Geometry check sheet. Reference: the model listing, model coordinates, mm. A direction names the side the tool comes from. Give positions to 0.01 mm unless a question says otherwise; leave off trailing zeros. Loops run counter-clockwise (first coordinate to the right, second up) from the corner with the lowest first, then second, coordinate; pieces in that order, holes last. Notation, with made-up numbers: (49, 36) -> (92, 36) arc R22 cw to (92, 72) -> close; hole circle Ø1 at (-6.5, 81). An arc over 180 degrees is marked (long way). One line per question, with ' | ' between items.
Autodesk Inventor part; units mm, degrees
ref_plane "YZ Plane" through (0, 0, 0) normal (1, 0, 0) x (0, 1, 0)
ref_plane "XZ Plane" through (0, 0, 0) normal (0, 1, 0) x (-1, 0, 0)
ref_plane "XY Plane" through (0, 0, 0) normal (0, 0, 1) x (1, 0, 0)
sketch "スケッチ1" plane through (0, 0, 0) normal (0, 0, 1) x (1, 0, 0)
  line L0 (-5, 5) -> (5, 5)
  line L1 (5, 5) -> (5, -5)
  line L2 (5, -5) -> (-5, -5)
  line L3 (-5, -5) -> (-5, 5)
  line L4 (-5, 5) -> (5, -5) construction
  line L5 (5, 5) -> (-5, -5) construction
  point P0 (0, 0)
  dimension "d0" = 10
  dimension "d1" = 10
extrude "押し出し1" add sketch "スケッチ1" along normal blind 1
sketch "スケッチ4" plane through (0, 0, 1) normal (0, 0, 1) x (1, 0, 0)
  line L0 (-5, 5) -> (5, 5)
  line L1 (5, 5) -> (5, 6)
  line L2 (5, 6) -> (-5, 6)
  line L3 (-5, 6) -> (-5, 5)
  point P0 (0, 0)
  dimension "d11" = 1
extrude "押し出し2" add sketch "スケッチ4" against normal blind 30
sketch "スケッチ9" plane through (0, 0, 0) normal (0, 0, -1) x (-1, 0, 0)
  line L0 (-5, -5) -> (5, -5)
  line L1 (5, -5) -> (5, 5)
  line L2 (5, 5) -> (-5, 5)
  line L3 (-5, 5) -> (-5, -5)
  point P0 (0, 0)
extrude "押し出し6" add sketch "スケッチ9" along normal blind 0.5
sketch "スケッチ10" plane through (0, 0, 1) normal (0, 0, 1) x (1, 0, 0)
  circle A0 centre (0, 0) radius 1.55
  dimension "d37" = 3.1
extrude "押し出し7" cut sketch "スケッチ10" against normal blind 3
sketch "スケッチ11" plane through (-5, 5, -29) normal (0, -1, 0) x (1, 0, 0)
  line L0 (0, 0) -> (10, 0)
  line L1 (10, 0) -> (10, 28.5)
  line L2 (10, 28.5) -> (0, 28.5)
  line L3 (0, 28.5) -> (0, 0)
  point P0 (5, 29)
extrude "押し出し8" add sketch "スケッチ11" along normal blind 0.5
sketch "スケッチ12" plane through (-5, 6, 1) normal (0, 1, 0) x (1, 0, 0)
  line L0 (10, 0) -> (10, 30)
  point P0 (5, 1)
  point P1 (5, 25)
  point P2 (5, 9)
  dimension "d42" = 16
  dimension "d43" = 8
  dimension "d44" = 5
hole "穴3" at (0, 6, -24) at (0, 6, -8) direction (0, -1, 0) diameter 2.2 depth 8 tip angle 118
properties part number "Servo catch front" material "アルミニウム 1100-H14"
Item 1: Scan lines: probe 1 along Z at (x, y) = (0, 5.3); probe 2 along Y at (x, z) = (0, 0.75); probe 3 along X at (y, z) = (5.6, -24). Record each from-to range of solid material in increasing order.
Result:
probe 1: -29 to -25.1, -22.9 to -9.1, -6.9 to 1 | probe 2: -5 to -1.55, 1.55 to 6 | probe 3: -5 to -1.1, 1.1 to 5
Item 2: Sectioned sample at A-A (x = 0). Record the cut outline in (y, z), plus the area to 3 significant figures.
Result:
outline: (-5, -0.5) -> (-1.55, -0.5) -> (-1.55, 1) -> (-5, 1) -> close; (1.55, -0.5) -> (4.5, -0.5) -> (4.5, -6.9) -> (6, -6.9) -> (6, 1) -> (1.55, 1) -> close; (4.5, -29) -> (6, -29) -> (6, -25.1) -> (4.5, -25.1) -> close; (4.5, -22.9) -> (6, -22.9) -> (6, -9.1) -> (4.5, -9.1) -> close | area: 48.0 mm2
Item 3: Sectioned sample at D-D (x = 2.25). Record the cut outline in (y, z).
Result:
outline: (-5, -0.5) -> (4.5, -0.5) -> (4.5, -29) -> (6, -29) -> (6, 1) -> (-5, 1) -> close
Item 4: Depth check by flat-ended pin: pin 1 Ø2 at (x, z) = (0, -8) entering from +Y; pin 2 Ø3.5 at (x, z) = (0, -24) entering from -Y; pin 3 Ø4 at (x, y) = (0, 0) entering from -Z. Enter the tip coordinate at first touch or a pass-through.
Result:
pin 1: through | pin 2: y = 4.5 | pin 3: z = -0.5
Item 5: Sectioned sample at C-C (y = 0). Record the cut outline in (x, z), plus the area to 4 significant figures.
Result:
outline: (-5, -0.5) -> (-1.55, -0.5) -> (-1.55, 1) -> (-5, 1) -> close; (1.55, -0.5) -> (5, -0.5) -> (5, 1) -> (1.55, 1) -> close | area: 10.35 mm2
Item 6: Release check for a two-part mould opening along Z. For faces 3 (the face through (0, 5.2, -25.1)), 4 (the face through (0, 5, -29)), 5 (the face through (0.715, -1.375, 0.26)) record: pulls with the +Z half, pulls with the -Z half, needs draft (parallel to the pull), parting line crosses it, or undercut.
Result:
face 3: undercut | face 4: pulls with the -Z half | face 5: needs draft
Item 7: Set-up check for faces 1 (the face through (0, 4.5, -15)), 2 (the face through (0, -5, 0)): record each of +Z, -Z, +X, -X, +Y, -Y from which the full face is reachable in a straight line by a thin tool's end or side.
Result:
face 1: -Z, +X, -X, -Y | face 2: +Z, -Z, +X, -X, -Y
Item 8: Sectioned sample at B-B (z = -24). Record the cut outline in (x, y).
Result:
outline: (-5, 4.5) -> (-1.1, 4.5) -> (-1.1, 6) -> (-5, 6) -> close; (1.1, 4.5) -> (5, 4.5) -> (5, 6) -> (1.1, 6) -> close
